The listing builds one solid part. Answer for the finished solid, in the listing's coordinates (mm). Face numbers are marked on the shaded views. A direction names the side the tool comes from. Round coordinates to 2 decimals unless told otherwise and drop trailing zeros. Order: outer loops, then holes, each group sorted by start corner. A loop starts at its lowest first (then second) coordinate and runs counter-clockwise, first axis right, second up. Notation, with made-up numbers: (74, -20.5) -> (78, -20.5) arc R22 cw to (78, 16.5) -> close; hole circle Ø7 at (86.25, -17.75). An arc over 180 degrees is marked (long way). Return JSON: item names as keys, results as strings. Group by question number.
(1) Which of the six approach directions +Z, -Z, +X, -X, +Y, -Y give full straight-line access (tool end or side, diameter ignored) to the marked faces 4, 5, 6, 7 and 8?
(2) The part is cut by section D-D (x = 23.5). Determine the outline of the cut face in (y, z).
(3) The part is cut by section B-B (z = 0.9). Determine the outline of the cut face in (x, y), plus the area to 3 significant figures.
(4) Consider line 1 (X direction, y = 8.9, z = -23.2); line 2 (X direction, y = 3.25, z = -47.3); line 3 (Y direction, x = -1, z = -11). Determine where each line is inside the solid, lowest interval first. Write a range as [from, to].
(5) Each of these flat-tipped pins is pushed along its axis until it touches: pin 1 (3 mm diameter, centred on x = 38.3, z = -23.2, fed in from +Y); pin 2 (2 mm diameter, centred on x = 11, z = -7, fed in from +Y); pin 3 (2.5 mm diameter, centred on x = 36, y = -3, fed in from +Z). Where does it stop, or does it pass through?
(6) The part is cut by section C-C (z = -18.5). Determine the outline of the cut face in (x, y), plus the area to 3 significant figures.
(7) The part is cut by section A-A (x = 35.4). Determine the outline of the cut face in (y, z).
(8) Determine the mould class of the marked faces 1, 2 and 3 for opening direction X: +X half, -X half, draft (parallel to the pull), parting line (faces both ways), or undercut.
from build123d import *

# Parameters (mm, degrees)
SKETCH1_W           = 46.4
SKETCH1_H           = 5.9
SKETCH1_W_2         = 42.4
SKETCH1_H_2         = 3.5
BOSS_EXTRUDE1_DEPTH = 32.5
FILLET2_R           = 3
SKETCH2_W           = 54
SKETCH2_H           = 13.5
SKETCH2_W_2         = 42.4
SKETCH2_H_2         = 3.5
BOSS_EXTRUDE2_DEPTH = 5.8
SKETCH3_W           = 54
SKETCH3_H           = 13.5
SKETCH3_W_2         = 42.4
SKETCH3_H_2         = 3.5
BOSS_EXTRUDE3_DEPTH = 5.8
SKETCH4_R           = 1.6
CUT_EXTRUDE1_DEPTH  = 65.569187698
SKETCH8_R           = 4
BOSS_EXTRUDE4_DEPTH = 13.5
CUT_EXTRUDE4_DEPTH  = 4
SKETCH15_W          = 42.4
SKETCH15_H          = 3.5
SKETCH15_W_2        = 5.8
SKETCH15_H_2        = 2.88
CUT_EXTRUDE5_DEPTH  = 71.197863215
FILLET3_R           = 2


with BuildPart() as part:
    # Sketch1 → Boss-Extrude1 (new body)
    with BuildSketch(Plane(origin=(0, 0, 0), x_dir=(0, 0, -1), z_dir=(1, 0, 0))):
        with Locations((23.2, 2.95)):
            Rectangle(SKETCH1_W, SKETCH1_H)
        with Locations((23.2, 2.95)):
            Rectangle(SKETCH1_W_2, SKETCH1_H_2, mode=Mode.SUBTRACT)
    extrude(amount=BOSS_EXTRUDE1_DEPTH)

    # Fillet2
    # the kernel refuses this fillet: 3 mm, written as the material it takes off along each edge
    with BuildSketch(Plane(origin=(-7.5, 0, -46.4), x_dir=(0, 0, 1), z_dir=(1, 0, 0)), Plane(origin=(-7.5, 5.9, 0), x_dir=(0, 0, -1), z_dir=(1, 0, 0)), Plane(origin=(-7.5, 5.9, -46.4), x_dir=(0, -1, 0), z_dir=(1, 0, 0))) as fillet2_piece_1:
        with BuildLine():
            CenterArc((FILLET2_R, -FILLET2_R), FILLET2_R, 90, 90)
            Line((0, -FILLET2_R), (0, 0))
            Line((0, 0), (FILLET2_R, 0))
        make_face()
    extrude(amount=47.5, mode=Mode.SUBTRACT)
    with BuildSketch(Plane(origin=(-7.5, 0, 0), x_dir=(0, 0, -1), z_dir=(1, 0, 0))) as fillet2_piece_2:
        with BuildLine():
            CenterArc((FILLET2_R, FILLET2_R), FILLET2_R, 180, 90)
            Line((0, FILLET2_R), (0, 0))
            Line((0, 0), (FILLET2_R, 0))
        make_face()
    extrude(amount=47.5, mode=Mode.SUBTRACT)

    # Sketch2 → Boss-Extrude2 (add)
    with BuildSketch(Plane(origin=(32.5, 0, 0), x_dir=(0, 0, -1), z_dir=(1, 0, 0))):
        with Locations((23.2, 2.95)):
            Rectangle(SKETCH2_W, SKETCH2_H)
        with Locations((23.2, 2.95)):
            Rectangle(SKETCH2_W_2, SKETCH2_H_2, mode=Mode.SUBTRACT)
    extrude(amount=BOSS_EXTRUDE2_DEPTH)

    # Sketch3 → Boss-Extrude3 (add)
    with BuildSketch(Plane.ZY):
        with Locations((-23.2, 2.95)):
            Rectangle(SKETCH3_W, SKETCH3_H)
        with Locations((-23.2, 2.95)):
            Rectangle(SKETCH3_W_2, SKETCH3_H_2, mode=Mode.SUBTRACT)
    extrude(amount=BOSS_EXTRUDE3_DEPTH)

    # Sketch4 → Cut-Extrude1 (cut, through all)
    with BuildSketch(Plane(origin=(0, 9.7, 0), x_dir=(1, 0, 0), z_dir=(0, 1, 0))):
        with Locations(Location((-2.9, 47.3, 0), (0, 0, 270))):
            Circle(SKETCH4_R)
        with Locations(Location((35.4, 47.3, 0), (0, 0, 270))):
            Circle(SKETCH4_R)
        with Locations(Location((-2.9, -0.9, 0), (0, 0, 270))):
            Circle(SKETCH4_R)
        with Locations(Location((35.4, -0.9, 0), (0, 0, 270))):
            Circle(SKETCH4_R)
    extrude(amount=-CUT_EXTRUDE1_DEPTH, mode=Mode.SUBTRACT)

    # Sketch8 → Boss-Extrude4 (add)
    with BuildSketch(Plane(origin=(0, 9.7, 0), x_dir=(1, 0, 0), z_dir=(0, 1, 0))):
        with Locations(Location((38.3, 23.2, 0), (0, 0, 270))):
            Circle(SKETCH8_R)
    extrude(amount=-BOSS_EXTRUDE4_DEPTH)

    # Sketch13 → CSK for M2 Flat Head Machine Screw1 (revolve, cut)
    with BuildSketch(Plane(origin=(38.3, 9.7, -23.2), x_dir=(0, 0, 1), z_dir=(1, 0, 0))):
        Polygon((0, 0), (0, 13.5), (1, 13.5), (1, 3.75), (2, 2.75), (2, 0), align=None)
    revolve(axis=Axis((38.3, 16.05, -23.2), (0, -1, 0)), mode=Mode.SUBTRACT)

    # Sketch14 → Cut-Extrude4 (cut)
    with BuildSketch(Plane.XZ.offset(3.8)):
        Polygon((38.3, -20.775128869), (36.2, -21.987564435), (36.2, -24.412435565), (38.3, -25.624871131), (40.4, -24.412435565), (40.4, -21.987564435), align=None)
    extrude(amount=-CUT_EXTRUDE4_DEPTH, mode=Mode.SUBTRACT)

    # Sketch15 → Cut-Extrude5 (cut, through all)
    with BuildSketch(Plane.ZY.offset(5.8)):
        with Locations((-23.2, 2.95)):
            Rectangle(SKETCH15_W, SKETCH15_H)
        with Locations((-47.3, -2.36)):
            Rectangle(SKETCH15_W_2, SKETCH15_H_2)
        with Locations((0.9, -2.36)):
            Rectangle(SKETCH15_W_2, SKETCH15_H_2)
    extrude(amount=-CUT_EXTRUDE5_DEPTH, mode=Mode.SUBTRACT)

    # Fillet3
    fillet3_edges = [part.edges().sort_by_distance(p)[0] for p in [
        (-5.8, -3.8, -23.2),
    ]]
    fillet(fillet3_edges, radius=FILLET3_R)


solid = part.part
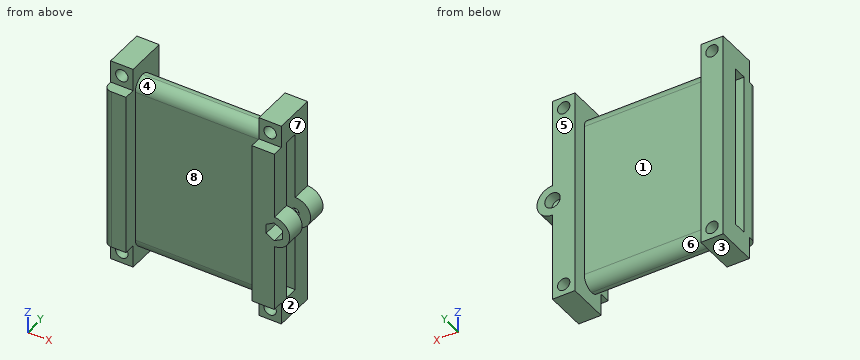
Answer below:
{
 "1": {"face 4": "+Z, -Y", "face 5": "+Z, -Z, +X, -X, +Y", "face 6": "-Z, +Y", "face 7": "+Z, +X, +Y, -Y", "face 8": "+Z, -Z, -Y"},
 "2": {"outline": "(0, -43.4) arc R3 ccw to (2.95, -46.4) arc R3 ccw to (5.9, -43.4) -> (5.9, -3) arc R3 ccw to (2.95, 0) arc R3 ccw to (0, -3) -> close; hole (1.2, -44.4) -> (4.7, -44.4) -> (4.7, -2) -> (1.2, -2) -> close"},
 "3": {"outline": "(-5.8, -0.92) -> (-4.5, -0.92) -> (-4.5, 9.7) -> (-5.8, 9.7) -> close; (-1.3, -0.92) -> (0, -0.92) -> (0, 9.7) -> (-1.3, 9.7) -> close; (32.5, -0.92) -> (33.8, -0.92) -> (33.8, 9.7) -> (32.5, 9.7) -> close; (37, -0.92) -> (38.3, -0.92) -> (38.3, 9.7) -> (37, 9.7) -> close", "area": "55.2 mm²"},
 "4": {"line 1": "x = [-5.8, 0], [32.5, 36.3], [40.3, 42.3]", "line 2": "x = [-5.8, -4.5], [-1.3, 0], [32.5, 33.8], [37, 38.3]", "line 3": "y = [-3.8, 1.2], [4.7, 9.7]"},
 "5": {"pin 1": "stops at y = 6.45", "pin 2": "stops at y = 5.9", "pin 3": "stops at z = -2"},
 "6": {"outline": "(-5.8, -1.8) arc R2 ccw to (-3.8, -3.8) -> (0, -3.8) -> (0, 0) -> (32.5, 0) -> (32.5, -3.8) -> (38.3, -3.8) -> (38.3, 1.2) -> (-5.8, 1.2) -> close; (-5.8, 4.7) -> (38.3, 4.7) -> (38.3, 9.7) -> (32.5, 9.7) -> (32.5, 5.9) -> (0, 5.9) -> (0, 9.7) -> (-5.8, 9.7) -> close", "area": "193 mm²"},
 "7": {"outline": "(-3.8, -44.4) -> (-0.92, -44.4) -> (-0.92, -45.7) -> (9.7, -45.7) -> (9.7, -0.7) -> (-0.92, -0.7) -> (-0.92, -2) -> (-3.8, -2) -> close; (-0.92, -50.2) -> (9.7, -50.2) -> (9.7, -48.9) -> (-0.92, -48.9) -> close; (-0.92, 2.5) -> (9.7, 2.5) -> (9.7, 3.8) -> (-0.92, 3.8) -> close; hole (1.2, -44.4) -> (4.7, -44.4) -> (4.7, -2) -> (1.2, -2) -> close"},
 "8": {"face 1": "undercut", "face 2": "+X half", "face 3": "draft"}
}
